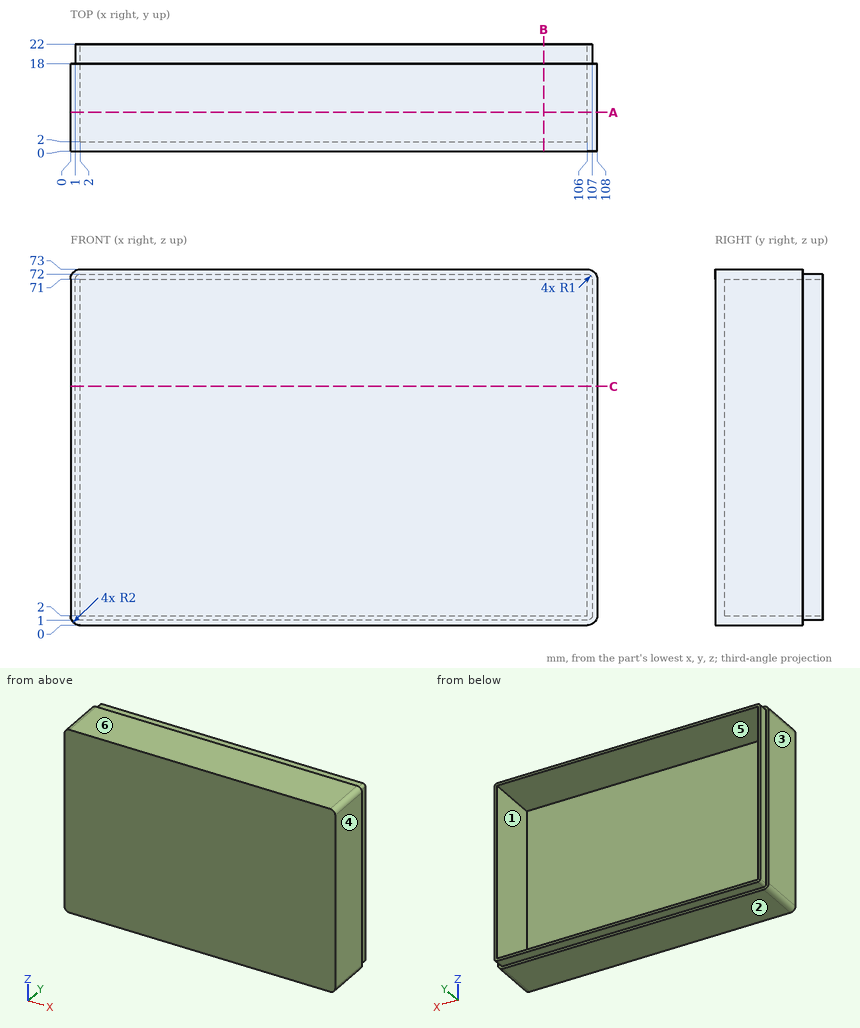
Study the drawing (mm; zero at the part's minimum x, y, z) and answer. A direction names the side the tool comes from. Round coordinates to 2 decimals unless told otherwise and drop trailing zeros. Write each loop counter-clockwise with the first axis right and the second up, starting at its lowest first coordinate (ties: lowest second). Pieces come first, ordered by that corner, then holes.
1) A cutting plane is placed at B-B (x = 97). Give the vertices of the cut face in (y, z).
2) The mould has two halves that part along X. Classify the marked faces 3, 4, 5 and 6: pulls with the +X half, pulls with the -X half, needs draft (parallel to the pull), parting line crosses it, or undercut.
3) A tool of negligible diameter and unlimited length cuts with its end or side. For the marked faces 1 and 2, from which of +Z, -Z, +X, -X, +Y, -Y can it reach the whole face along a straight path? Write none if from no direction.
4) A cutting plane is placed at C-C (z = 49). Give the vertices of the cut face in (x, y), plus the area to 3 significant figures.
5) A cutting plane is placed at A-A (y = 8). Give the vertices of the cut face in (x, z), plus the area to 3 significant figures.
6) Given pin 1 Ø1.2 at (x, y) = (61, 19.5) entering from -Z; pin 2 Ø5 at (x, z) = (51, 44.5) entering from +Y; pin 3 Ø1.2 at (x, y) = (74.5, 19) entering from +Z, each flat-ended and moving along its own axis, determine where each tip first touches the part or whether it passes through.
7) Straight lines are drawn through the part: line 1 (Z direction, x = 77, y = 8.75); line 2 (Z direction, x = 42.5, y = 21.25); line 3 (X direction, y = 3.5, z = 28.5). For each, find the intervals that lie inside material, in ascending order.
Completed:
1. outline: (0, 0) - (18, 0) - (18, 1) - (22, 1) - (22, 2) - (2, 2) - (2, 71) - (22, 71) - (22, 72) - (18, 72) - (18, 73) - (0, 73) - close
2. face 3: pulls with the -X half
2. face 4: pulls with the +X half
2. face 5: undercut
2. face 6: needs draft
3. face 1: +Y
3. face 2: -Z, +X, -X, +Y, -Y
4. outline: (0, 0) - (108, 0) - (108, 18) - (107, 18) - (107, 22) - (106, 22) - (106, 2) - (2, 2) - (2, 22) - (1, 22) - (1, 18) - (0, 18) - close
4. area: 288 mm2
5. outline: (0, 2) arc R2 ccw to (2, 0) - (106, 0) arc R2 ccw to (108, 2) - (108, 71) arc R2 ccw to (106, 73) - (2, 73) arc R2 ccw to (0, 71) - close; hole (2, 2) - (106, 2) - (106, 71) - (2, 71) - close
5. area: 705 mm2
6. pin 1: stops at z = 1
6. pin 2: stops at y = 2
6. pin 3: stops at z = 72
7. line 1: z = 0 to 2, 71 to 73
7. line 2: z = 1 to 2, 71 to 72
7. line 3: x = 0 to 2, 106 to 108
